Input: part model. Units: mm. Frame: model coordinates. Face numbers are marked on the shaded views. A direction names the side the tool comes from. Round coordinates to 2 decimals unless told otherwise and drop trailing zeros. Loops run counter-clockwise (first coordinate to the right, second up) from the corner with the lowest first, then second, coordinate; pieces in that order, holes last.
(1) Cut plane A-A, the plane x = 0. Output: boundary loops of the cut face in (y, z) (3 decimals), and give its area (3 significant figures).
(2) Cut plane D-D, the plane z = -1.75. Output: boundary loops of the cut face in (x, y), and give its area (3 significant figures).
(3) First-contact query: pin 1 Ø1.5 at (y, z) = (4.5, -2) entering from +X; pin 2 Ø3 at (x, z) = (1, 2.5) entering from -Y; pin 3 Ø1.5 at (y, z) = (2.5, 1) entering from +X; pin 4 Ø1.6 at (x, z) = (0, 0) entering from +Y. Flat tips, straight axial feed; report the tip coordinate or a pass-through.
(4) Line query: line 1 (Z direction, x = 0, y = 5.75) (3 decimals); line 2 (Z direction, x = 0, y = 10.25); line 3 (Y direction, x = -2.25, z = 1.75). Output: solid intervals per line, ascending.
(5) Draft query along X for the marked faces 1, 2 and 3. Return one class per face: released by +X, released by -X, zero draft, split by the parting line, or undercut.
(6) Cut plane C-C, the plane y = 5.5. Output: boundary loops of the cut face in (x, z) (3 decimals).
(7) Cut plane B-B, the plane z = 0. Output: boundary loops of the cut face in (x, y) (3 decimals).
(8) Access query for the marked faces 4, 5 and 6. Directions: +Z, -Z, +X, -X, +Y, -Y. A direction counts if a zero-diameter tool reaches every point of the face in a straight line with its end or side. Return the directions, or none.
Autodesk Inventor part; units mm, degrees
ref_plane "YZ Plane" through (0, 0, 0) normal (1, 0, 0) x (0, 1, 0)
ref_plane "XZ Plane" through (0, 0, 0) normal (0, 1, 0) x (-1, 0, 0)
ref_plane "XY Plane" through (0, 0, 0) normal (0, 0, 1) x (1, 0, 0)
sketch "Sketch2" plane through (0, 0, 0) normal (0, 1, 0) x (-1, 0, 0)
  circle A0 centre (0, 0) radius 3
  dimension "d0" = 6
extrude "Extrusion1" add sketch "Sketch2" along normal blind 5
sketch "Sketch3" plane through (0, 5, 0) normal (0, 1, 0) x (1, 0, 0)
  circle A0 centre (0, 0) radius 1.475
  dimension "d3" = 2.95
extrude "Extrusion2" add sketch "Sketch3" along normal blind 2.1
sketch "Sketch4" plane through (0, 7.1, 0) normal (0, 1, 0) x (1, 0, 0)
  circle A0 centre (0, 0) radius 3.5
  dimension "d6" = 7
extrude "Extrusion3" add sketch "Sketch4" along normal blind 10
sketch "Sketch5" plane through (0, 17.1, 0) normal (0, 1, 0) x (1, 0, 0)
  point P0 (0, 0)
  point P1 (0, 0)
hole "Hole1" at (0, 17.1, 0) direction (0, -1, 0) diameter 2 end through all
thread "Thread1"
thread "Thread2"
properties part number "Chimera Heatbreak" material "Aluminum 6061, Welded"
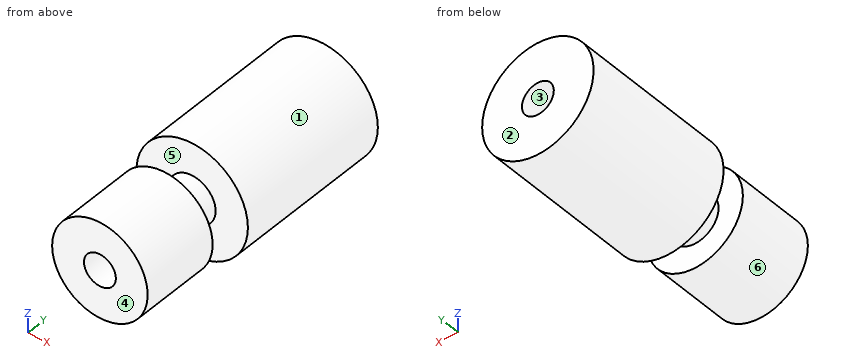
Reported:
1. outline: (0, -3) - (5, -3) - (5, -1.475) - (7.1, -1.475) - (7.1, -3.5) - (17.1, -3.5) - (17.1, -1) - (0, -1) - close; (0, 1) - (17.1, 1) - (17.1, 3.5) - (7.1, 3.5) - (7.1, 1.475) - (5, 1.475) - (5, 3) - (0, 3) - close
1. area: 72.0 mm2
2. outline: (-3.03, 7.1) - (3.03, 7.1) - (3.03, 17.1) - (-3.03, 17.1) - close; (-2.44, 0) - (2.44, 0) - (2.44, 5) - (-2.44, 5) - close
2. area: 85.0 mm2
3. pin 1: stops at x = 2.73
3. pin 2: stops at y = 0
3. pin 3: stops at x = 2.99
3. pin 4: passes through
4. line 1: z = -1.475 to -1, 1 to 1.475
4. line 2: z = -3.5 to -1, 1 to 3.5
4. line 3: y = 0 to 5, 7.1 to 17.1
5. face 1: split by the parting line
5. face 2: zero draft
5. face 3: undercut
6. outline: circle Ø2.95 at (0, 0); hole circle Ø2 at (0, 0)
7. outline: (-3.5, 7.1) - (-1.475, 7.1) - (-1.475, 5) - (-3, 5) - (-3, 0) - (-1, 0) - (-1, 17.1) - (-3.5, 17.1) - close; (1, 0) - (3, 0) - (3, 5) - (1.475, 5) - (1.475, 7.1) - (3.5, 7.1) - (3.5, 17.1) - (1, 17.1) - close
8. face 4: +Z, -Z, +X, -X, -Y
8. face 5: none
8. face 6: -Y
